from build123d import *

# Parameters (mm, degrees)
BOSS_EXTRUDE1_START = 710
SKETCH2_W           = 616.707969139
SKETCH2_H           = 579.165034538
BOSS_EXTRUDE1_DEPTH = 483
SKETCH3_W           = 594.672235047
SKETCH3_H           = 426.228299924
CUT_EXTRUDE1_DEPTH  = 568
CUT_EXTRUDE2_START  = -100
CUT_EXTRUDE2_DEPTH  = 23


with BuildPart() as part:
    # Sketch2 → Boss-Extrude1 (new body)
    with BuildSketch(Plane.XY.offset(943.510776168).offset(BOSS_EXTRUDE1_START)):
        with Locations((826.513525673, 479.417482731)):
            Rectangle(SKETCH2_W, SKETCH2_H)
    extrude(amount=BOSS_EXTRUDE1_DEPTH)

    # Sketch3 → Cut-Extrude1 (cut)
    with BuildSketch(Plane(origin=(0, 769, 0), x_dir=(1, 0, 0), z_dir=(0, 1, 0))):
        with Locations((827.567040516, -1907.628066077)):
            Rectangle(SKETCH3_W, SKETCH3_H)
    extrude(amount=-CUT_EXTRUDE1_DEPTH, mode=Mode.SUBTRACT)

    # Sketch4 → Cut-Extrude2 (cut)
    with BuildSketch(Plane(origin=(0, 769, 0), x_dir=(1, 0, 0), z_dir=(0, 1, 0)).offset(CUT_EXTRUDE2_START)):
        with BuildLine():
            Line((826.513525672, -1680.127363582), (826.513525672, -1653.510776168))
            Line((826.513525672, -1653.510776168), (882.617138286, -1653.510776168))
            ThreePointArc((882.617138286, -1653.510776168), (858.584109748, -1675.290026262), (826.513525672, -1680.127363582))
        make_face()
    extrude(amount=-CUT_EXTRUDE2_DEPTH, mode=Mode.SUBTRACT)


solid = part.part
The listing builds one solid part. Answer for the finished solid, in the listing's coordinates (mm). A direction names the side the tool comes from. Give positions to 0.01 mm unless a question says otherwise; leave off trailing zeros. Order: outer loops, then holes, each group sorted by start corner. A loop starts at its lowest first (then second) coordinate and runs counter-clockwise, first axis right, second up. Notation, with made-up numbers: (58, -28.5) - (114, -28.5) arc R15 cw to (114, -2.5) - close; hole circle Ø7 at (54.5, 5.5). An arc over 180 degrees is marked (long way). One line per item, written item: value. Start each with the question number.
1) The mould has two halves that part along Z. Classify faces 4 (the face through (530.231, 489, 1911)), 5 (the face through (1134.868, 475, 1892)), 6 (the face through (822, 483, 2136.511)): released by +Z, released by -Z, zero draft, split by the parting line, or undercut.
2) A tool of negligible diameter and unlimited length cuts with its end or side. For faces 1 (the face through (849, 646, 1664)), 2 (the face through (823, 489, 2120.742)), 3 (the face through (734, 769, 1679)), from which of +Z, -Z, +X, -X, +Y, -Y can it reach the whole face along a straight path? Write none if from no direction.
3) A cutting plane is placed at A-A on y = 616.5. Give the vertices of the cut face in (x, z), then the cut area to 3 significant figures.
4) Given pin 1 Ø6 at (x, z) = (607.5, 1950.5) entering from +Y, flat-ended and moving along its own axis, determine where the tip first touches the part or whether it passes through.
5) A cutting plane is placed at B-B on z = 2097. Give the vertices of the cut face in (x, y).
6) Find the intervals of material crossed by L1, parallel to Z at x = 788, y = 252.5; L2, parallel to X at y = 669.5, z = 1701; L3, parallel to Y at x = 750, z = 1755, in increasing order.
7) A cutting plane is placed at C-C on x = 596.5. Give the vertices of the cut face in (y, z), then the cut area to 3 significant figures.
Answer sheet:
1. face 4: undercut
1. face 5: zero draft
1. face 6: released by +Z
2. face 1: -Z
2. face 2: +Y
2. face 3: +Z, -Z, +X, -X, +Y
3. outline: (518.16, 1653.51) - (1134.87, 1653.51) - (1134.87, 2136.51) - (518.16, 2136.51) - close; hole (530.23, 1694.51) - (1124.9, 1694.51) - (1124.9, 2120.74) - (530.23, 2120.74) - close
3. area: 44,400 mm2
4. pin 1: stops at y = 201
5. outline: (518.16, 189.83) - (1134.87, 189.83) - (1134.87, 769) - (1124.9, 769) - (1124.9, 201) - (530.23, 201) - (530.23, 769) - (518.16, 769) - close
6. L1: z = 1653.51 to 1694.51, 2120.74 to 2136.51
6. L2: x = 518.16 to 530.23, 1124.9 to 1134.87
6. L3: y = 189.83 to 201
7. outline: (189.83, 1653.51) - (769, 1653.51) - (769, 1694.51) - (201, 1694.51) - (201, 2120.74) - (769, 2120.74) - (769, 2136.51) - (189.83, 2136.51) - close
7. area: 37,600 mm2
